Verification items for the finished model (mm, model axes). A direction names the side the tool comes from. Give positions to 0.01 mm unless a question says otherwise; leave off trailing zeros. Loops run counter-clockwise (first coordinate to the right, second up) from the corner with the lowest first, then second, coordinate; pieces in that order, holes last. Notation, with made-up numbers: (-20, 26) - (2, 26) arc R24 ccw to (2, 43) - close; hole circle Ø2 at (0, 59). An arc over 180 degrees is marked (long way). One line per item, written item: value. Start each with the question number.
1. Sectioned sample at A-A (z = 1.5). Record the cut outline in (x, y).
2. Sectioned sample at C-C (y = -19). Record the cut outline in (x, z).
3. Access from +Z, -Z, +X, -X, +Y, -Y to the whole of each face (thin tool, end or side, straight path). Record for faces 1 (the flat face through (-34, 14.56, 0)), 2 (the flat face through (-38, 4.56, 0)), 3 (the flat face through (-80, 10, 3)).
4. Sectioned sample at B-B (x = -74). Record the cut outline in (y, z).
5. Scan lines: L1, parallel to Y at x = -73, z = 0; L2, parallel to Y at x = 63, z = -0.25. Record each from-to range of solid material in increasing order. Write a range as [from, to].
6. Gauge pin test, flat ends, axial feed: pin 1 (4 mm diameter, centred on x = 20, z = 1.5, fed in from -Y); pin 2 (3 mm diameter, centred on y = 7, z = -0.5, fed in from -X). Record the tip position at first contact, or that the pin passes through.
7. Mould release check, pull along Z, two halves, no side actions. Record for faces 4 (the cylindrical face through (-82.08, 7.34, 3.49)), 5 (the flat face through (19, 1, -4)), 6 (the flat face through (-77.231, 9, 0)), 7 (the flat face through (19, 1, 4)): pulls with the +Z half, pulls with the -Z half, needs draft (parallel to the pull), parting line crosses it, or undercut.
from build123d import *

# Parameters (mm, degrees)
SKETCH_1_R          = 2.5
SKETCH_1_R_2        = 1.5
EXTRUDE_2_DEPTH     = 4
CUT_EXTRUDE_1_DEPTH = 3


with BuildPart() as part:
    # 草图1 → 凸台-拉伸2 (new, symmetric)
    with BuildSketch(Plane.XY):
        with BuildLine():
            Line((-83.231357553, 14.560229446), (-43.231357553, 14.560229446))
            Line((-43.231357553, 14.560229446), (16.768642447, 14.560229446))
            Line((16.768642447, 14.560229446), (109.865069812, -21.95079919))
            Line((109.865069812, -21.95079919), (90.555427075, -28.299696326))
            Line((90.555427075, -28.299696326), (6.768642447, 4.560229446))
            Line((6.768642447, 4.560229446), (-43.231357553, 4.560229446))
            Line((-43.231357553, 4.560229446), (-83.231357553, 4.560229446))
            ThreePointArc((-83.231357553, 4.560229446), (-88.231357553, 9.560229446), (-83.231357553, 14.560229446))
        make_face()
        with Locations((-83.231357553, 9.560229446)):
            Circle(SKETCH_1_R, mode=Mode.SUBTRACT)
        with Locations((13.041147127, 9.560229446)):
            Circle(SKETCH_1_R_2, mode=Mode.SUBTRACT)
    extrude(amount=EXTRUDE_2_DEPTH, both=True)

    # 草图2 → 切除-拉伸1 (cut, symmetric)
    with BuildSketch(Plane.XY):
        with BuildLine():
            Line((-83.231357553, 4.560229446), (-77.231357553, 4.560229446))
            Line((-77.231357553, 4.560229446), (-77.231357553, 14.560229446))
            Line((-77.231357553, 14.560229446), (-83.231357553, 14.560229446))
            ThreePointArc((-83.231357553, 14.560229446), (-88.231357553, 9.560229446), (-83.231357553, 4.560229446))
        make_face()
    extrude(amount=CUT_EXTRUDE_1_DEPTH, both=True, mode=Mode.SUBTRACT)


solid = part.part
Results are:
1. outline: (-77.23, 4.56) - (6.77, 4.56) - (90.56, -28.3) - (109.87, -21.95) - (16.77, 14.56) - (-77.23, 14.56) - close; hole circle Ø3 at (13.04, 9.56)
2. outline: (66.84, -4) - (102.34, -4) - (102.34, 4) - (66.84, 4) - close
3. face 1: +Z, -Z, +X, -X, +Y
3. face 2: +Z, -Z, -X, -Y
3. face 3: -X, +Y, -Y
4. outline: (4.56, -4) - (14.56, -4) - (14.56, 4) - (4.56, 4) - close
5. L1: y = [4.56, 14.56]
5. L2: y = [-17.49, -3.57]
6. pin 1: stops at y = -1.41
6. pin 2: stops at x = -77.23
7. face 4: needs draft
7. face 5: pulls with the -Z half
7. face 6: undercut
7. face 7: pulls with the +Z half
